```python
from build123d import *


# Not quite as in the source:
# - a feature names something its author has since deleted; it is built from what else it names


with BuildPart() as f1:
    # F0 (on Front) → F1 (revolve)
    with BuildSketch(Plane.XZ):
        with BuildLine():
            Line((22.3186584817, 4.9634656969), (15.2303930372, 1.2544910423))
            Line((15.2303930372, 1.2544910423), (15.488850391, 0.9470738952))
            Line((15.488850391, 0.9470738952), (15.5328564546, 0.894731726))
            Line((15.5328564546, 0.894731726), (15.8405525238, 1.0429841968))
            Line((15.8405525238, 1.0429841968), (22.4313864066, 4.2185444515))
            ThreePointArc((22.4313864066, 4.2185444515), (24.744105662, 3.4097946744), (23.9353558848, 1.097075419))
            Line((23.9353558848, 1.097075419), (16.3696151821, 0.4137007552))
            Line((16.3696151821, 0.4137007552), (15.9677918852, 0.3774061119))
            Line((15.9677918852, 0.3774061119), (16.2850916386, 0))
            Line((16.2850916386, 0), (24.2850916386, 0))
            ThreePointArc((24.2850916386, 0), (25.023915829, 0.2087553322), (25.5442474517, 0.7732860891))
            Line((25.5442474517, 0.7732860891), (25.5442474517, 4.3952541752))
            ThreePointArc((25.5442474517, 4.3952541752), (24.028202675, 5.2285828576), (22.3186584817, 4.9634656969))
        make_face()
        Polygon((15.8405525238, 1.0429841968), (15.5328564546, 0.894731726), (15.9677918852, 0.3774061119), (16.3696151821, 0.4137007552), align=None)
    revolve(axis=Axis((0, 0, 1.8443568842), (0, 0, 1)))

    # F2 (on Front) → F3 (revolve)
    with BuildSketch(Plane.XZ):
        Polygon((-25.3970567137, 3.7070766557), (-28.3970567137, 3.7070766557), (-28.3970567137, 4.2962685693), (-30.5454257131, 3.7070766557), (-30.5454257131, 3.2924627885), (-25.5454257131, 3.2924627885), align=None)
    revolve(axis=Axis((-26.2971473858, 0, 2.2924627885), (-1, 0, 0)))


solid = f1.part
```
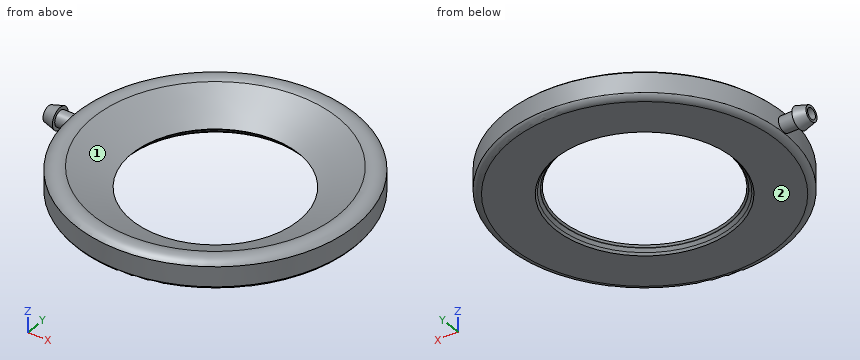
Verification items for the finished model (mm, model axes). Face numbers are marked on the shaded views. Give positions to 0.01 mm unless a question says otherwise; leave off trailing zeros. One line per question, with ' | ' between items.
Item 1: Draft check along X on the marked faces 1 and 2. Enter one of: +X half, -X half, draft (parallel to the pull), parting line (faces both ways), or undercut.
Completed:
face 1: undercut | face 2: draft
Item 2: Depth check by flat-ended pin: P1, Ø2, axis at y = 2, z = 2.5, coming from the +X side; P2, Ø2, axis at x = -3, z = 4, coming from the -Y side; P3, Ø2, axis at x = -6.5, z = 0.5, coming from the -Y side. Enter the tip coordinate at first touch or a pass-through.
Completed:
P1: stops at x = 25.52 | P2: stops at y = -25.47 | P3: stops at y = -24.94
Item 3: Section check A-A, the plane z = 2.6. State how many separate pieces and enclosed holes the cut face has, plus the area to 3 significant figures.
Completed:
separate pieces: 2 | enclosed holes: 2 | area: 253 mm^2
Item 4: Thickness scan on line 1 (X direction, y = 3, z = 2.3); line 2 (Y direction, x = 5, z = 3.1); line 3 (Y direction, x = 5, z = 3.4). Record the ranges inside material, lowest first. Write a range as [from, to].
Completed:
line 1: x = [-25.37, -24.7], [-18.2, -16.97], [16.97, 18.2], [24.7, 25.37] | line 2: y = [-25.05, -24.35], [-19.48, -18.08], [18.08, 19.48], [24.35, 25.05] | line 3: y = [-25.05, -24.24], [-20.12, -18.67], [18.67, 20.12], [24.24, 25.05]
